from build123d import *

# Parameters (mm, degrees)
SKETCH1_W           = 15.088
SKETCH1_H           = 15.088
SKETCH1_R           = 4.4
BOSS_EXTRUDE1_DEPTH = 235


with BuildPart() as part:
    # Sketch1 → Boss-Extrude1 (new, symmetric)
    # profile 1 of 5: a face of its own
    with BuildSketch(Plane.XY):
        with BuildLine():
            Line((-7.544, 7.544), (-5.784718328, 7.544))
            Line((-5.784718328, 7.544), (-11.512, 13.271281672))
            Line((-11.512, 13.271281672), (-11.512, 16.8))
            Line((-11.512, 16.8), (-6.051976926, 16.8))
            Line((-6.051976926, 16.8), (-9.251976926, 20))
            Line((-9.251976926, 20), (-17, 20))
            ThreePointArc((-17, 20), (-19.121320344, 19.121320344), (-20, 17))
            Line((-20, 17), (-20, 9.251976926))
            Line((-20, 9.251976926), (-16.8, 6.051976926))
            Line((-16.8, 6.051976926), (-16.8, 11.512))
            Line((-16.8, 11.512), (-13.271281672, 11.512))
            Line((-13.271281672, 11.512), (-7.544, 5.784718328))
            Line((-7.544, 5.784718328), (-7.544, 7.544))
        make_face()
    # profile 2 of 5: a face of its own
    with BuildSketch(Plane.XY):
        with BuildLine():
            Line((11.512, 13.271281672), (5.784718328, 7.544))
            Line((5.784718328, 7.544), (7.544, 7.544))
            Line((7.544, 7.544), (7.544, 5.784718328))
            Line((7.544, 5.784718328), (13.271281672, 11.512))
            Line((13.271281672, 11.512), (16.8, 11.512))
            Line((16.8, 11.512), (16.8, 6.051976926))
            Line((16.8, 6.051976926), (20, 9.251976926))
            Line((20, 9.251976926), (20, 17))
            ThreePointArc((20, 17), (19.121320344, 19.121320344), (17, 20))
            Line((17, 20), (9.251976926, 20))
            Line((9.251976926, 20), (6.051976926, 16.8))
            Line((6.051976926, 16.8), (11.512, 16.8))
            Line((11.512, 16.8), (11.512, 13.271281672))
        make_face()
    # profile 3 of 5: a face of its own
    with BuildSketch(Plane.XY):
        with BuildLine():
            Line((-7.544, -7.544), (-7.544, -5.784718328))
            Line((-7.544, -5.784718328), (-13.271281672, -11.512))
            Line((-13.271281672, -11.512), (-16.8, -11.512))
            Line((-16.8, -11.512), (-16.8, -6.051976926))
            Line((-16.8, -6.051976926), (-20, -9.251976926))
            Line((-20, -9.251976926), (-20, -17))
            ThreePointArc((-20, -17), (-19.121320344, -19.121320344), (-17, -20))
            Line((-17, -20), (-9.251976926, -20))
            Line((-9.251976926, -20), (-6.051976926, -16.8))
            Line((-6.051976926, -16.8), (-11.512, -16.8))
            Line((-11.512, -16.8), (-11.512, -13.271281672))
            Line((-11.512, -13.271281672), (-5.784718328, -7.544))
            Line((-5.784718328, -7.544), (-7.544, -7.544))
        make_face()
    # profile 4 of 5: a face of its own
    with BuildSketch(Plane.XY):
        with BuildLine():
            Line((13.271281672, -11.512), (7.544, -5.784718328))
            Line((7.544, -5.784718328), (7.544, -7.544))
            Line((7.544, -7.544), (5.784718328, -7.544))
            Line((5.784718328, -7.544), (11.512, -13.271281672))
            Line((11.512, -13.271281672), (11.512, -16.8))
            Line((11.512, -16.8), (6.051976926, -16.8))
            Line((6.051976926, -16.8), (9.251976926, -20))
            Line((9.251976926, -20), (17, -20))
            ThreePointArc((17, -20), (19.121320344, -19.121320344), (20, -17))
            Line((20, -17), (20, -9.251976926))
            Line((20, -9.251976926), (16.8, -6.051976926))
            Line((16.8, -6.051976926), (16.8, -11.512))
            Line((16.8, -11.512), (13.271281672, -11.512))
        make_face()
    # profile 5 of 5: a face of its own
    with BuildSketch(Plane.XY):
        Rectangle(SKETCH1_W, SKETCH1_H)
        with Locations(Location((0, 0, 0), (0, 0, 180))):
            Circle(SKETCH1_R, mode=Mode.SUBTRACT)
    extrude(amount=BOSS_EXTRUDE1_DEPTH, both=True)


solid = part.part
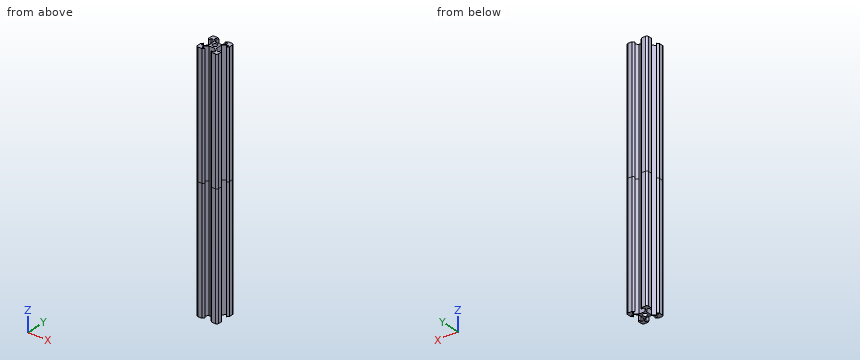
Input: part model. Units: mm. Frame: model coordinates. Coordinates: 2 decimals unless noted, no trailing zeros. Loops run counter-clockwise (first coordinate to the right, second up) from the corner with the lowest first, then second, coordinate; pieces in that order, holes last. Notation, with made-up numbers: (-11, 51) -> (22, 51) arc R29 cw to (22, 71) -> close; hole circle Ø8 at (-0.75, 20.5). An arc over 180 degrees is marked (long way). Write each question's results on one line, items separated by ' | '. Start each with the question number.
Q1. Section A-A, the plane y = 0. Return the cut outline in (x, z), plus the area to 3 significant figures.
Q2. Ray query, line 1 (X direction, y = 14.5, z = -71.5); line 2 (Y direction, x = 0, z = 180.5); line 3 (Y direction, x = -11, z = -170). Return the intervals inside material, ascending. Write a range as from..to.
Q3. Pin query (flat end, axial travel): pin 1 (1 mm diameter, centred on x = 8, z = 6.5, fed in from -Y); pin 2 (5.5 mm diameter, centred on x = 0, y = 0, fed in from -Z); pin 3 (1.6 mm diameter, centred on y = 8, z = 145, fed in from +X). Return the tip coordinate at first contact, or that it passes through.
Found:
1) outline: (-7.54, -235) -> (-4.4, -235) -> (-4.4, 235) -> (-7.54, 235) -> close; (4.4, -235) -> (7.54, -235) -> (7.54, 235) -> (4.4, 235) -> close | area: 2,960 mm2
2) line 1: -20..-11.51, 11.51..20 | line 2: -7.54..-4.4, 4.4..7.54 | line 3: -20..-16.8, -12.76..-9.24, 9.24..12.76, 16.8..20
3) pin 1: y = -19.25 | pin 2: through | pin 3: x = 19.55
